```python
from build123d import *

# Parameters (mm, degrees)
F0_W     = 53
F0_H     = 5
F0_R     = 12.5
F0_W_2   = 48
F1_DEPTH = 5


with BuildPart() as f1:
    # F0 (on Right) → F1 (new body)
    with BuildSketch(Plane.YZ):
        with Locations((98.5, -52.5)):
            Rectangle(F0_W, F0_H)
        Polygon((72, -50), (125, -50), (125, 0), (120, 0), (120, 50), (5, 50), (5, 40), (0, 40), (-5, 40), (-5, 50), (-120, 50), (-120, 0), (-125, 0), (-125, -50), (-72, -50), (-24, -50), (24, -50), align=None)
        Circle(F0_R, mode=Mode.SUBTRACT)
        with Locations((0, -52.5)):
            Rectangle(F0_W_2, F0_H)
        with Locations((-98.5, -52.5)):
            Rectangle(F0_W, F0_H)
    extrude(amount=F1_DEPTH)


solid = f1.part
```
For this review, take the finished solid that the model builds, in its own axes (mm). A direction names the side the tool comes from. Give positions to 0.01 mm unless a question says otherwise; leave off trailing zeros. Write each loop counter-clockwise with the first axis right and the second up, starting at its lowest first coordinate (ties: lowest second). Pieces come first, ordered by that corner, then holes.
Item 1: Take a section at D-D (y = -40.5). Give the boundary of the cut face in (x, z), and give its area (3 significant figures).
Item 2: Machinability: for faces 1 (the face through (2, 120, 25)), 2 (the face through (2, -5, 45)), 3 (the face through (2, -72, -53)), which of the approach directions +Z, -Z, +X, -X, +Y, -Y give a long, thin tool a straight path to every point of the face, cutting with its end or side? Answer none if there is none.
Item 3: Wall thickness on probe 1 along Z at (x, y) = (2.95, 0); probe 2 along Y at (x, z) = (1.15, 22); probe 3 along Y at (x, z) = (4.1, -5): over which ranges is each line inside the solid? List them lowest first.
Item 4: Insertion check: P1, Ø2.5, axis at x = 2.5, y = -123.5, coming from the +Z side; P2, Ø2.5, axis at x = 2.5, z = 45, coming from the +Y side; P3, Ø1.5, axis at x = 2, y = -38.5, coming from the -Z side. Each pin has a flat end and moves straight along its axis. Give the tip position at first contact, or say it passes through.
Item 5: Take a section at B-B (x = 3.25). Give the boundary of the cut face in (y, z), and give its area (3 significant figures).
Item 6: Take a section at A-A (y = 0). Give the boundary of the cut face in (x, z).
Item 7: Take a section at C-C (z = 34). Give the boundary of the cut face in (x, y).
Established:
1. outline: (0, -50) - (5, -50) - (5, 50) - (0, 50) - close
1. area: 500 mm2
2. face 1: +Z, +X, -X, +Y
2. face 2: +Z, +X, -X
2. face 3: -Z, +X, -X
3. probe 1: z = -55 to -12.5, 12.5 to 40
3. probe 2: y = -120 to 120
3. probe 3: y = -125 to -11.46, 11.46 to 125
4. P1: stops at z = 0
4. P2: stops at y = 120
4. P3: stops at z = -50
5. outline: (-125, -55) - (-72, -55) - (-72, -50) - (-24, -50) - (-24, -55) - (24, -55) - (24, -50) - (72, -50) - (72, -55) - (125, -55) - (125, 0) - (120, 0) - (120, 50) - (5, 50) - (5, 40) - (-5, 40) - (-5, 50) - (-120, 50) - (-120, 0) - (-125, 0) - close; hole circle Ø25 at (0, 0)
5. area: 24,700 mm2
6. outline: (0, -55) - (5, -55) - (5, -12.5) - (0, -12.5) - close; (0, 12.5) - (5, 12.5) - (5, 40) - (0, 40) - close
7. outline: (0, -120) - (5, -120) - (5, 120) - (0, 120) - close
